Geometry check sheet. Reference: drawing and pictorial views, mm from the part's lowest x, y, z. A direction names the side the tool comes from. Give positions to 0.01 mm unless a question says otherwise; leave off trailing zeros. Write each loop counter-clockwise with the first axis right and the second up, starting at its lowest first coordinate (ties: lowest second). Pieces come first, ordered by that corner, then holes.
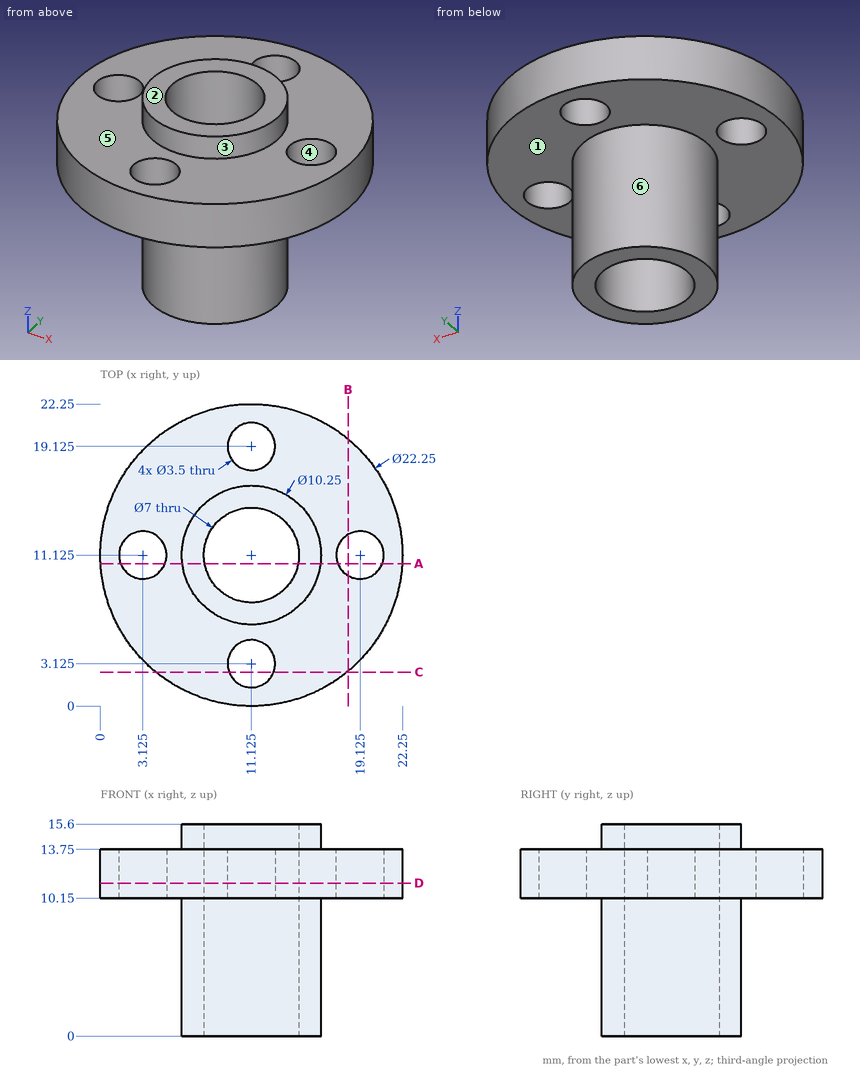
Item 1: Set-up check for the marked faces 1, 2 and 3: record each of +Z, -Z, +X, -X, +Y, -Y from which the full face is reachable in a straight line by a thin tool's end or side.
Answer key:
face 1: -Z
face 2: +Z, +X, -X, +Y, -Y
face 3: +Z
Item 2: Sectioned sample at C-C on y = 2.5. Record the cut outline in (x, z).
Answer key:
outline: (4.1, 10.15) - (9.49, 10.15) - (9.49, 13.75) - (4.1, 13.75) - close; (12.76, 10.15) - (18.15, 10.15) - (18.15, 13.75) - (12.76, 13.75) - close
Item 3: Scan lines: line 1 along Y through (x, z) = (11, 4.25); line 2 along Z through (x, y) = (3.5, 13); line 3 along Y through (x, z) = (9, 13). Record each from-to range of solid material in increasing order.
Answer key:
line 1: y = 6 to 7.63, 14.62 to 16.25
line 2: z = 10.15 to 13.75
line 3: y = 0.2 to 8.34, 13.91 to 22.05
Item 4: Sectioned sample at A-A on y = 10.5. Record the cut outline in (x, z), then the cut area to 3 significant figures.
Answer key:
outline: (0.02, 10.15) - (1.49, 10.15) - (1.49, 13.75) - (0.02, 13.75) - close; (4.76, 10.15) - (6.04, 10.15) - (6.04, 0) - (7.68, 0) - (7.68, 15.6) - (6.04, 15.6) - (6.04, 13.75) - (4.76, 13.75) - close; (14.57, 0) - (16.21, 0) - (16.21, 10.15) - (17.49, 10.15) - (17.49, 13.75) - (16.21, 13.75) - (16.21, 15.6) - (14.57, 15.6) - close; (20.76, 10.15) - (22.23, 10.15) - (22.23, 13.75) - (20.76, 13.75) - close
area: 71.1 mm2
Item 5: Sectioned sample at D-D on z = 11.25. Record the cut outline in (x, y) (3 decimals).
Answer key:
outline: circle Ø22.25 at (11.125, 11.125); hole circle Ø3.5 at (3.125, 11.125); hole circle Ø7 at (11.125, 11.125); hole circle Ø3.5 at (11.125, 3.125); hole circle Ø3.5 at (11.125, 19.125); hole circle Ø3.5 at (19.125, 11.125)
Item 6: Release check for a two-part mould opening along X. For the marked faces 4, 5 and 6 record: released by +X, released by -X, zero draft, split by the parting line, or undercut.
Answer key:
face 4: undercut
face 5: zero draft
face 6: split by the parting line
Item 7: Depth check by flat-ended pin: pin 1 (1 mm diameter, centred on y = 15, z = 12, fed in from -X); pin 2 (6 mm diameter, centred on x = 15, z = 2, fed in from -Y); pin 3 (5.5 mm diameter, centred on x = 11.125, y = 19.125, fed in from +Z); pin 4 (3 mm diameter, centred on x = 11.125, y = 3.125, fed in from +Z). Enter the tip coordinate at first touch or a pass-through.
Answer key:
pin 1: stops at x = 0.52
pin 2: stops at y = 6.08
pin 3: stops at z = 13.75
pin 4: passes through
Item 8: Sectioned sample at B-B on x = 18.25. Record the cut outline in (y, z).
Answer key:
outline: (2.58, 10.15) - (9.61, 10.15) - (9.61, 13.75) - (2.58, 13.75) - close; (12.64, 10.15) - (19.67, 10.15) - (19.67, 13.75) - (12.64, 13.75) - close
